```python
from build123d import *

# Parameters (mm, degrees)
BOSS_EXTRUDE1_DEPTH = 7
SKETCH2_R           = 50
SKETCH2_W           = 6.441902201
SKETCH2_H           = 3
SKETCH2_W_2         = 5.266935295
CUT_EXTRUDE1_DEPTH  = 37.691279618
FILLET1_R           = 2
FILLET2_R           = 1.5


with BuildPart() as part:
    # Sketch1 → Boss-Extrude1 (new body)
    with BuildSketch(Plane.XY):
        with BuildLine():
            Line((0, 0), (12.5, 0))
            ThreePointArc((12.5, 0), (17.5, 5), (22.5, 0))
            Line((22.5, 0), (35, 0))
            Line((35, 0), (35, 8.5))
            Line((35, 8.5), (0, 8.5))
            Line((0, 8.5), (0, 0))
        make_face()
    extrude(amount=BOSS_EXTRUDE1_DEPTH)

    # Sketch2 → Cut-Extrude1 (cut, through all)
    with BuildSketch(Plane(origin=(0, 8.5, 0), x_dir=(1, 0, 0), z_dir=(0, 1, 0))):
        with Locations((17.5, 48)):
            Circle(SKETCH2_R)
        with Locations((17.5, -55)):
            Circle(SKETCH2_R)
        with Locations((37.220951101, -3.5)):
            Rectangle(SKETCH2_W, SKETCH2_H)
        with Locations((-1.633467648, -3.5)):
            Rectangle(SKETCH2_W_2, SKETCH2_H)
    extrude(amount=-CUT_EXTRUDE1_DEPTH, mode=Mode.SUBTRACT)

    # Fillet1
    fillet1_edges = [part.edges().sort_by_distance(p)[0] for p in [
        (35, 4.25, 0),
        (35, 4.25, 7),
        (0, 4.25, 7),
        (0, 4.25, 0),
        (1, 0, 3.5),
        (34, 0, 3.5),
    ]]
    fillet(fillet1_edges, radius=FILLET1_R - 0.0001)  # a hair under: the kernel refuses the full size

    # Fillet2
    fillet2_edges = [part.edges().sort_by_distance(p)[0] for p in [
        (17.48803644, 4.999985682, 1.999998553),
        (17.48803647, 4.999985682, 5.000001447),
    ]]
    fillet(fillet2_edges, radius=FILLET2_R - 0.0001)  # a hair under: the kernel refuses the full size


solid = part.part
```
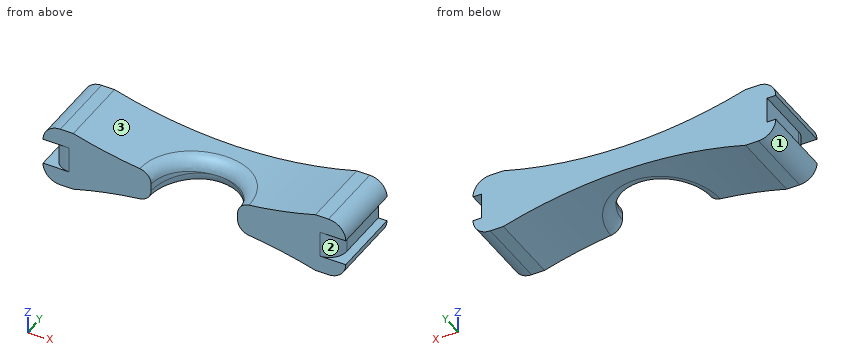
Verification items for the finished model (mm, model axes). Face numbers are marked on the shaded views. Coordinates: 2 decimals unless noted, no trailing zeros. Loops run counter-clockwise (first coordinate to the right, second up) from the corner with the lowest first, then second, coordinate; pieces in that order, holes last. Notation, with made-up numbers: (-14, 60.5) - (30, 60.5) arc R22 cw to (30, 67.5) - close; hole circle Ø7 at (-30.75, -39.5). An arc over 180 degrees is marked (long way). Answer as a JSON object with one key per item and string values.
(1) Cross-section at B-B, the plane x = 9. Record the boundary of the cut face in (y, z).
Response:
{"outline": "(0, 1.27) - (8.5, 1.27) - (8.5, 5.73) - (0, 5.73) - close"}
(2) Mould release check, pull along X, two halves, no side actions. Record for the marked faces 1, 2 and 3: pulls with the +X half, pulls with the -X half, needs draft (parallel to the pull), parting line crosses it, or undercut.
Response:
{"face 1": "pulls with the -X half", "face 2": "pulls with the +X half", "face 3": "undercut"}
(3) Go/stop test with flat-tipped pins: pin 1 Ø1.5 at (x, z) = (26, 1) entering from +Y; pin 2 Ø0.9 at (y, z) = (4.5, 3) entering from +X; pin 3 Ø5 at (x, y) = (14.5, 5) entering from +Z. Record where each tip stops, or that it passes through.
Response:
{"pin 1": "stops at y = 8.5", "pin 2": "stops at x = 34", "pin 3": "stops at z = 5.3"}
(4) Cross-section at A-A, the plane z = 1. Record the boundary of the cut face in (x, y).
Response:
{"outline": "(0.27, 0) - (7.55, 0) - (7.55, 8.5) - (0.27, 8.5) - close; (27.45, 0) - (34.73, 0) - (34.73, 8.5) - (27.45, 8.5) - close"}
(5) Scan lines: line 1 along X through (y, z) = (2.25, 3); line 2 along X through (y, z) = (5.5, 4.5); line 3 along X through (y, z) = (3, 3.25). Record each from-to range of solid material in increasing order.
Response:
{"line 1": "x = 1 to 13.02, 21.98 to 34", "line 2": "x = 1 to 34", "line 3": "x = 1 to 13.5, 21.5 to 34"}
